The model under review builds one solid part; all positions refer to its coordinate system, in mm. A direction names the side the tool comes from. Give positions to 0.01 mm unless a question says otherwise; leave off trailing zeros. Loops run counter-clockwise (first coordinate to the right, second up) from the corner with the lowest first, then second, coordinate; pieces in that order, holes last. Notation, with made-up numbers: (35, 45) - (70, 45) arc R16 cw to (70, 70) - close; hole circle Ø9 at (20, -39.5). An arc over 180 degrees is marked (long way). Answer as a JSON object with one key per item and string values.
from build123d import *

# Parameters (mm, degrees)
SKETCH10_W          = 150
SKETCH10_H          = 150
BOSS_EXTRUDE3_DEPTH = 10
SKETCH12_W          = 100
SKETCH12_H          = 37.5
CUT_EXTRUDE2_DEPTH  = 10
FILLET7_R           = 10
CUT_EXTRUDE3_DEPTH  = 35


with BuildPart() as part:
    # Sketch10 → Boss-Extrude3 (new body)
    with BuildSketch(Plane(origin=(0, 0, 0), x_dir=(0, 0, -1), z_dir=(1, 0, 0))):
        with Locations((75, 112.5)):
            Rectangle(SKETCH10_W, SKETCH10_H)
    extrude(amount=BOSS_EXTRUDE3_DEPTH)

    # Sketch12 → Cut-Extrude2 (cut)
    with BuildSketch(Plane.ZY):
        with Locations((-75, 56.25)):
            Rectangle(SKETCH12_W, SKETCH12_H)
    extrude(amount=-CUT_EXTRUDE2_DEPTH, mode=Mode.SUBTRACT)

    # Fillet7
    fillet7_edges = [part.edges().sort_by_distance(p)[0] for p in [
        (5, 37.5, -125),
        (5, 37.5, -25),
        (5, 187.5, 0),
        (5, 187.5, -150),
        (5, 37.5, -150),
        (5, 37.5, 0),
    ]]
    fillet(fillet7_edges, radius=FILLET7_R)

    # Sketch13 → Cut-Extrude3 (cut)
    with BuildSketch(Plane(origin=(10, 0, 0), x_dir=(0, 0, -1), z_dir=(1, 0, 0))):
        with BuildLine():
            Line((50, 177.5), (100, 177.5))
            ThreePointArc((100, 177.5), (107.5, 170), (100, 162.5))
            Line((100, 162.5), (50, 162.5))
            ThreePointArc((50, 162.5), (42.5, 170), (50, 177.5))
        make_face()
    extrude(amount=-CUT_EXTRUDE3_DEPTH, mode=Mode.SUBTRACT)


solid = part.part
Q1. Consider section B-B, the plane y = 170. State the section outline as (x, z) points, plus the area to 3 significant figures.
Results:
{"outline": "(0, -150) - (10, -150) - (10, -107.5) - (0, -107.5) - close; (0, -42.5) - (10, -42.5) - (10, 0) - (0, 0) - close", "area": "850 mm^2"}
Q2. Clearance check with a flat-ended pin moving along its axis: pin 1 Ø5 at (x, z) = (4, -99) entering from -Y. State where the tip first meets the part, or that it passes through.
Results:
{"pin 1": "stops at y = 75"}
Q3. For faces 1 (the face through (5.07, 170.16, -107.5)), 2 (the face through (5, 61, -125)), 3 (the face through (10, 114, -74)), list the 3-axis set-ups (+Z, -Z, +X, -X, +Y, -Y) from which the entire face can be reached by the end or side of a thin tool; tool diameter is ignored.
Results:
{"face 1": "+X, -X", "face 2": "+X, -X, -Y", "face 3": "+Z, -Z, +X, +Y, -Y"}
Q4. The part is to be moulded in two halves that separate along Y. For faces 4 (the face through (5.07, 40.35, -128.01)), 5 (the face through (5.07, 184.49, -2.85)), 6 (the face through (5.07, 169.84, -42.5)), say which applies: +Y half, -Y half, draft (parallel to the pull), parting line (faces both ways), or undercut.
Results:
{"face 4": "-Y half", "face 5": "+Y half", "face 6": "undercut"}
Q5. Consider section A-A, the plane x = 7. State the section outline as (y, z) points.
Results:
{"outline": "(37.5, -140) arc R10 ccw to (47.5, -150) - (177.5, -150) arc R10 ccw to (187.5, -140) - (187.5, -10) arc R10 ccw to (177.5, 0) - (47.5, 0) arc R10 ccw to (37.5, -10) - (37.5, -15) arc R10 ccw to (47.5, -25) - (75, -25) - (75, -125) - (47.5, -125) arc R10 ccw to (37.5, -135) - close; hole (162.5, -100) arc R7.5 ccw to (177.5, -100) - (177.5, -50) arc R7.5 ccw to (162.5, -50) - close"}
Q6. To check wall thickness, follow probe 1 along Y at (x, z) = (0.5, -82.5); probe 2 along Z at (x, y) = (5, 72); probe 3 along Y at (x, z) = (9, -104.5). State the ranges of each line that lie inside material, in increasing order. Write a range as [from, to].
Results:
{"probe 1": "y = [75, 162.5], [177.5, 187.5]", "probe 2": "z = [-150, -125], [-25, 0]", "probe 3": "y = [75, 164], [176, 187.5]"}
